Build history of the part. All positions in model axes, mm. A direction names the side the tool comes from. Round coordinates to 2 decimals unless told otherwise and drop trailing zeros. Loops run counter-clockwise (first coordinate to the right, second up) from the corner with the lowest first, then second, coordinate; pieces in that order, holes last.
from build123d import *

# Parameters (mm, degrees)
SKETCH1_W            = 85.725
SKETCH1_H            = 50.8
BOSS_EXTRUDE1_DEPTH  = 6.35
SKETCH2_W            = 15.875
SKETCH2_H            = 43.18
CUT_EXTRUDE1_DEPTH   = 6.35
SKETCH3_W            = 85.725
SKETCH3_H            = 6.35
CUT_EXTRUDE2_DEPTH   = 0.762
SKETCH5_W            = 6.35
SKETCH5_H            = 6.35
CUT_EXTRUDE3_DEPTH   = 4.7625
SKETCH7_W            = 6.35
SKETCH7_H            = 6.858
CUT_EXTRUDE5_DEPTH   = 11.43
SKETCH8_W            = 53.975
SKETCH8_H            = 6.35
CUT_EXTRUDE6_DEPTH   = 6.35
M6_CLEARANCE_HOLE1_D = 7
SKETCH12_W           = 5.1689
SKETCH12_H           = 6.7564
CUT_EXTRUDE7_DEPTH   = 41.439530169


with BuildPart() as part:
    # Sketch1 → Boss-Extrude1 (new body)
    with BuildSketch(Plane.XY):
        Rectangle(SKETCH1_W, SKETCH1_H)
    extrude(amount=BOSS_EXTRUDE1_DEPTH)

    # Sketch2 → Cut-Extrude1 (cut)
    with BuildSketch(Plane.XY.offset(6.35)):
        with Locations((-34.925, -3.81)):
            Rectangle(SKETCH2_W, SKETCH2_H)
        with Locations((34.925, -3.81)):
            Rectangle(SKETCH2_W, SKETCH2_H)
    extrude(amount=-CUT_EXTRUDE1_DEPTH, mode=Mode.SUBTRACT)

    # Sketch3 → Cut-Extrude2 (cut)
    with BuildSketch(Plane(origin=(0, 25.4, 0), x_dir=(1, 0, 0), z_dir=(0, 1, 0))):
        with Locations((0, -3.175)):
            Rectangle(SKETCH3_W, SKETCH3_H)
    extrude(amount=-CUT_EXTRUDE2_DEPTH, mode=Mode.SUBTRACT)

    # Sketch5 → Cut-Extrude3 (cut)
    with BuildSketch(Plane.ZY.offset(26.9875)):
        with Locations((3.175, 14.605)):
            Rectangle(SKETCH5_W, SKETCH5_H)
    cut_extrude3 = extrude(amount=-CUT_EXTRUDE3_DEPTH, mode=Mode.SUBTRACT)

    # Mirror1: Cut-Extrude3 across plane
    add(cut_extrude3.mirror(Plane(origin=(0, 0, 0), x_dir=(0, 0, 1), z_dir=(1, 0, 0))), mode=Mode.SUBTRACT)

    # Sketch7 → Cut-Extrude5 (cut)
    with BuildSketch(Plane.ZY.offset(42.8625)):
        with Locations((3.175, 21.209)):
            Rectangle(SKETCH7_W, SKETCH7_H)
    cut_extrude5 = extrude(amount=-CUT_EXTRUDE5_DEPTH, mode=Mode.SUBTRACT)

    # Mirror2: Cut-Extrude5 across plane
    add(cut_extrude5.mirror(Plane(origin=(0, 0, 0), x_dir=(0, 0, 1), z_dir=(1, 0, 0))), mode=Mode.SUBTRACT)

    # Sketch8 → Cut-Extrude6 (cut)
    with BuildSketch(Plane.XZ.offset(25.4)):
        with Locations((0, 3.175)):
            Rectangle(SKETCH8_W, SKETCH8_H)
    extrude(amount=-CUT_EXTRUDE6_DEPTH, mode=Mode.SUBTRACT)

    # M6 Clearance Hole1 (through all)
    with Locations(Plane.XY.offset(6.35)):
        with Locations((0.00592, -7.666260004)):
            Hole(M6_CLEARANCE_HOLE1_D / 2)

    # Sketch12 → Cut-Extrude7 (cut, through all)
    with BuildSketch(Plane.XY.offset(6.35)):
        with Locations((-24.60625, 14.605)):
            Rectangle(SKETCH12_W, SKETCH12_H)
        with Locations((24.60625, 14.605)):
            Rectangle(SKETCH12_W, SKETCH12_H)
    extrude(amount=-CUT_EXTRUDE7_DEPTH, mode=Mode.SUBTRACT)


solid = part.part
(1) Slice it at A-A on y = -5. List the corners of the cut face in (x, z).
Responses:
outline: (-26.99, 0) - (-2.26, 0) - (-2.26, 6.35) - (-26.99, 6.35) - close; (2.27, 0) - (26.99, 0) - (26.99, 6.35) - (2.27, 6.35) - close
(2) Pull direction X, two halves, no side cores. Call faces 1 (the face through (0, 3, 0)), 2 (the face through (31.432, 21, 3)), 3 (the face through (0.5, -4.2, 3.1)): +X half, -X half, draft (parallel to the pull), parting line (faces both ways), or undercut.
Responses:
face 1: draft
face 2: +X half
face 3: undercut
(3) Probe line 1 (Y direction, x = 0, z = 3.5); line 2 (Y direction, x = -26, z = 2.25); line 3 (X direction, y = -17, z = 0.75). List the from-to ranges inside material, lowest first.
Responses:
line 1: y = -19.05 to -11.17, -4.17 to 24.64
line 2: y = -19.05 to 11.23, 17.98 to 24.64
line 3: x = -26.99 to 26.99
(4) Slice it at C-C on y = 16.5. List the corners of the cut face in (x, z).
Responses:
outline: (-22.02, 0) - (22.02, 0) - (22.02, 6.35) - (-22.02, 6.35) - close
(5) Slice it at B-B on z = 1.25. List the corners of the cut face in (x, y), plus the area to 3 significant figures.
Responses:
outline: (-31.43, 17.78) - (-27.19, 17.78) - (-27.19, 17.98) - (-22.02, 17.98) - (-22.02, 11.23) - (-26.99, 11.23) - (-26.99, -19.05) - (26.99, -19.05) - (26.99, 11.23) - (22.02, 11.23) - (22.02, 17.98) - (27.19, 17.98) - (27.19, 17.78) - (31.43, 17.78) - (31.43, 24.64) - (-31.43, 24.64) - close; hole circle Ø7 at (0.01, -7.67)
area: 2,310 mm2
(6) Which spindle directions (+Z, -Z, +X, -X, +Y, -Y) get a long thin tool onto all of the face, cutting with end or side? Do faces 4 (the face through (25, 17.983, 3)), 5 (the face through (-29, 17.78, 3)), 6 (the face through (29, 17.78, 3)). Say none if no direction does.
Responses:
face 4: +Z, -Z
face 5: +Z, -Z, -X, -Y
face 6: +Z, -Z, +X, -Y
(7) Slice it at D-D on y = 7. List the corners of the cut face in (x, z), plus the area to 3 significant figures.
Responses:
outline: (-26.99, 0) - (26.99, 0) - (26.99, 6.35) - (-26.99, 6.35) - close
area: 343 mm2
(8) Pin check, flat tips, straight feed: P1, Ø1.3, axis at x = -30, z = 1.5, coming from the -Y side; P2, Ø1.9, axis at y = 15, z = 4.5, coming from the -X side; P3, Ø1.9, axis at y = -3.5, z = 2, coming from the -X side. Stop position of each tip, or through.
Responses:
P1: stops at y = 17.78
P2: stops at x = -22.02
P3: stops at x = -26.99
